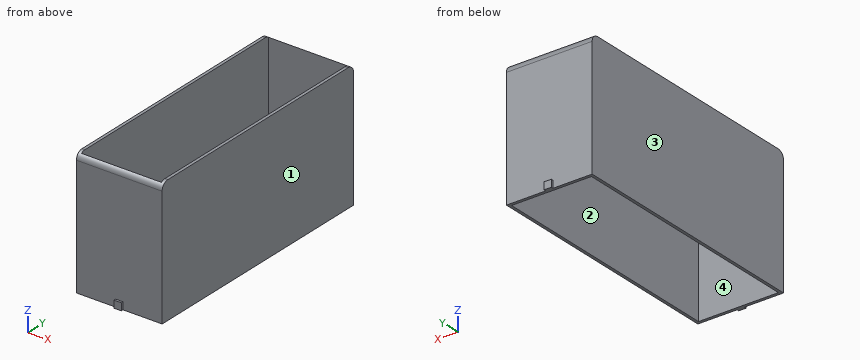
```python
from build123d import *

# Parameters (mm, degrees)
F0_W        = 23.6
F0_H        = 69
F0_W_2      = 22
F0_H_2      = 67.4
F1_DEPTH    = 35
F2_T1_DEPTH = 33.6
F3_W        = 2
F3_H        = 0.6
F4_DEPTH    = 2


# Not quite as in the source:
# - a fillet or chamfer that OpenCascade refuses, or shapes differently, is made with other operations: its cross-section is extruded or revolved along the edge and cut away or added


with BuildPart() as f1:
    # F0 (on Top) → F1 (new body)
    with BuildSketch(Plane.XY):
        Rectangle(F0_W, F0_H)
        Rectangle(F0_W_2, F0_H_2, mode=Mode.SUBTRACT)
    extrude(amount=F1_DEPTH)

    # F2: fillet of radius 2 on 2 edges, made by hand

    # F2_s2 → F2_t1 (cut)
    with BuildSketch(Plane.YZ.offset(-16.8)):
        with BuildLine():
            ThreePointArc((-34.5, 33), (-33.9142135624, 34.4142135624), (-32.5, 35))
            Line((-32.5, 35), (-34.5, 35))
            Line((-34.5, 35), (-34.5, 33))
        make_face()
        with BuildLine():
            ThreePointArc((34.5, 33), (33.9142135624, 34.4142135624), (32.5, 35))
            Line((32.5, 35), (34.5, 35))
            Line((34.5, 35), (34.5, 33))
        make_face()
    extrude(amount=F2_T1_DEPTH, mode=Mode.SUBTRACT)

    # F3 (on face) → F4 (join)
    with BuildSketch(Plane(origin=(0, 0, 0), x_dir=(1, 0, 0), z_dir=(0, 0, -1))):
        with Locations((0, 34.8)):
            Rectangle(F3_W, F3_H)
        with Locations((0, -34.8)):
            Rectangle(F3_W, F3_H)
    extrude(amount=-F4_DEPTH)


solid = f1.part
```
For this review, take the finished solid that the model builds, in its own axes (mm). Face numbers are marked on the shaded views. A direction names the side the tool comes from. Round coordinates to 2 decimals unless told otherwise and drop trailing zeros. Write each loop counter-clockwise with the first axis right and the second up, starting at its lowest first coordinate (ties: lowest second). Pieces come first, ordered by that corner, then holes.
1) Insertion check: pin 1 Ø1.5 at (x, z) = (-7, 8.5) entering from +Y; pin 2 Ø0.7 at (y, z) = (-35, 0.5) entering from +X; pin 3 Ø1 at (x, z) = (1, 8.5) entering from -Y. Each pin has a flat end and moves straight along its axis. Give the tip position at first contact, or say it passes through.
Answer below:
pin 1: stops at y = 34.5
pin 2: stops at x = 1
pin 3: stops at y = -34.5
2) Take a section at C-C on x = -8.5. Give the boundary of the cut face in (y, z).
Answer below:
outline: (-34.5, 0) - (-33.7, 0) - (-33.7, 34.6) arc R2 ccw to (-34.5, 33) - close; (33.7, 0) - (34.5, 0) - (34.5, 33) arc R2 ccw to (33.7, 34.6) - close
3) Take a section at A-A on z = 11.5. Give the boundary of the cut face in (x, y).
Answer below:
outline: (-11.8, -34.5) - (11.8, -34.5) - (11.8, 34.5) - (-11.8, 34.5) - close; hole (-11, -33.7) - (11, -33.7) - (11, 33.7) - (-11, 33.7) - close
4) Machinability: for the marked faces 1 and 2, which of the approach directions +Z, -Z, +X, -X, +Y, -Y give a long, thin tool a straight path to every point of the face, cutting with its end or side? Answer none if there is none.
Answer below:
face 1: +Z, -Z, +X, +Y, -Y
face 2: +Z, -Z
5) For line 1 along Y through (x, z) = (3.75, 5.5); line 2 along X through (y, z) = (-30.5, 6), list the stretches that pass through material, from the lowest coordinate up.
Answer below:
line 1: y = -34.5 to -33.7, 33.7 to 34.5
line 2: x = -11.8 to -11, 11 to 11.8
6) Mouldability with a two-part tool opening along Y and no side actions: class the marked faces 3 and 4 as +Y half, -Y half, draft (parallel to the pull), parting line (faces both ways), or undercut.
Answer below:
face 3: draft
face 4: undercut
7) Take a section at B-B on y = 9. Give the boundary of the cut face in (x, z).
Answer below:
outline: (-11.8, 0) - (-11, 0) - (-11, 35) - (-11.8, 35) - close; (11, 0) - (11.8, 0) - (11.8, 35) - (11, 35) - close
